Can you work these out from the model? Positions are in its coordinate system, mm. A direction names the side the tool comes from. Give positions to 0.01 mm unless a question says otherwise; leave off trailing zeros. Order: outer loops, then holes, each group sorted by start corner. A loop starts at its lowest first (then second) coordinate and runs counter-clockwise, first axis right, second up. Notation, with made-up numbers: M 88.25,10 L 97.25,10 A17 cw 97.25,20 Z; hole C -33,44 d4. An arc over 180 degrees is marked long. Answer as a JSON object with one key per item and string values.
```python
from build123d import *

# Parameters (mm, degrees)
F0_W     = 38.1
F0_H     = 12.7
F1_DEPTH = 368.3
F2_W     = 7.62
F2_H     = 6.35
F3_DEPTH = 368.301
F4_W     = 9.525
F4_H     = 12.7
F5_DEPTH = 25.4


with BuildPart() as f1:
    # F0 (on Front) → F1 (new body)
    with BuildSketch(Plane.XZ):
        with Locations((19.05, 6.35)):
            Rectangle(F0_W, F0_H)
    extrude(amount=F1_DEPTH)

    # F2 (on face) → F3 (cut, through all)
    with BuildSketch(Plane.XZ.offset(368.3)):
        with Locations((13.335, 3.175)):
            Rectangle(F2_W, F2_H)
    extrude(amount=-F3_DEPTH, mode=Mode.SUBTRACT)

    # F4 (on face) → F5 (cut)
    with BuildSketch(Plane.XY.offset(12.7)):
        with Locations((23.8125, -6.35)):
            Rectangle(F4_W, F4_H)
        with Locations((4.7625, -6.35)):
            Rectangle(F4_W, F4_H)
        with Locations((4.7625, -361.95)):
            Rectangle(F4_W, F4_H)
        with Locations((23.8125, -361.95)):
            Rectangle(F4_W, F4_H)
    extrude(amount=-F5_DEPTH, mode=Mode.SUBTRACT)


solid = f1.part
```
1) Thinking about a two-plate mould opening in X: for faces 5 (the face through (0, -182, 6)), 6 (the face through (5, -355.6, 6)), 7 (the face through (28.575, -6, 6)), which applies, pulls with the +X half, pulls with the -X half, needs draft (parallel to the pull), parting line crosses it, or undercut?
Results found:
{"face 5": "pulls with the -X half", "face 6": "needs draft", "face 7": "undercut"}
2) For faces 1 (the face through (9.525, -362, 10)), 2 (the face through (17.145, -187, 3)), 3 (the face through (24, -12.7, 6)), 4 (the face through (9.525, -6, 10)), which set-ups out of +Z, -Z, +X, -X, +Y, -Y let a thin tool reach every point of the face, with its end or its side?
Results found:
{"face 1": "+Z, -Z, -X, -Y", "face 2": "-Z, +Y, -Y", "face 3": "+Z, -Z, +Y", "face 4": "+Z, -Z, -X, +Y"}
3) I need wall thicknesses on L1, parallel to X at y = -314, z = 5.25 (3 decimals); L2, parallel to Z at x = 15, y = -161.5; L3, parallel to Y at x = 3, z = 8.75. Which ranges of each line are inside material? Lowest first, please.
Results found:
{"L1": "x = 0 to 9.525, 17.145 to 38.1", "L2": "z = 6.35 to 12.7", "L3": "y = -355.6 to -12.7"}
4) I want a section at B-B on y = -266. Write out the boundary of the cut face in (x, z) (3 decimals), and give its area (3 significant figures).
Results found:
{"outline": "M 0,0 L 9.525,0 L 9.525,6.35 L 17.145,6.35 L 17.145,0 L 38.1,0 L 38.1,12.7 L 0,12.7 Z", "area": "435 mm²"}
5) I want a section at C-C on x = 12.5. Write out the boundary of the cut face in (y, z).
Results found:
{"outline": "M -368.3,6.35 L 0,6.35 L 0,12.7 L -368.3,12.7 Z"}
6) I want a section at A-A on z = 2.25. Write out the boundary of the cut face in (x, y) (3 decimals), and give its area (3 significant figures).
Results found:
{"outline": "M 0,-355.6 L 9.525,-355.6 L 9.525,-12.7 L 0,-12.7 Z; M 17.145,-368.3 L 19.05,-368.3 L 19.05,-355.6 L 28.575,-355.6 L 28.575,-368.3 L 38.1,-368.3 L 38.1,0 L 28.575,0 L 28.575,-12.7 L 19.05,-12.7 L 19.05,0 L 17.145,0 Z", "area": "10,700 mm²"}
7) I'm going to push flat-ended pins straight in: pin 1 Ø4 at (x, y) = (13, -239.5) entering from -Z; pin 2 Ø1.9 at (y, z) = (-365, 8.5) entering from -X (3 decimals); pin 3 Ø3 at (x, z) = (4, 4) entering from -Y. Where does each tip first touch, or does it pass through?
Results found:
{"pin 1": "stops at z = 6.35", "pin 2": "stops at x = 9.525", "pin 3": "stops at y = -355.6"}
